The model under review builds one solid part; all positions refer to its coordinate system, in mm. Face numbers are marked on the shaded views. Give positions to 0.01 mm unless a question says otherwise; leave off trailing zeros. Loops run counter-clockwise (first coordinate to the right, second up) from the corner with the lowest first, then second, coordinate; pieces in that order, holes last. Notation, with made-up numbers: M 88.25,-9.75 L 128.25,-9.75 A25 ccw 128.25,20.25 Z; hole C 33.5,53 d10. An arc over 180 degrees is marked long. Return JSON: item names as keys, results as strings.
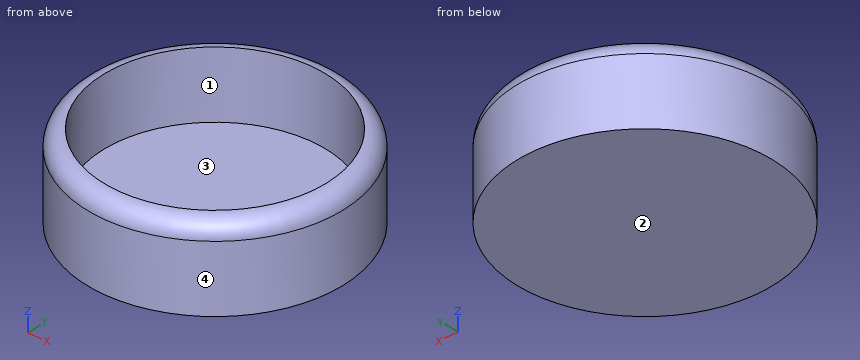
```python
from build123d import *

# Parameters (mm, degrees)
F0_R     = 23
F0_R_2   = 20
F1_DEPTH = 15
F2_R     = 23
F3_DEPTH = 3
F4_R     = 2.99999


# Not quite as in the source:
# - a fillet or chamfer is up to 0.001 mm smaller than in the source, because OpenCascade refuses the exact size


with BuildPart() as f1:
    # F0 (on Top) → F1 (new body)
    with BuildSketch(Plane.XY):
        Circle(F0_R)
        Circle(F0_R_2, mode=Mode.SUBTRACT)
    extrude(amount=F1_DEPTH)

    # F2 (on Top) → F3 (join)
    with BuildSketch(Plane.XY):
        Circle(F2_R)
    extrude(amount=F3_DEPTH)

    # F4 (radius 3 in the source; OpenCascade refuses exactly that, so slightly less here)
    f4_edges = [f1.edges().sort_by_distance(p)[0] for p in [
        (-23, 0, 15),
    ]]
    fillet(f4_edges, radius=F4_R)


solid = f1.part
```
1) Consider section C-C on z = 10.5. Write out the cut boundary in (x, y).
From the geometry:
{"outline": "C 0,0 d46; hole C 0,0 d40"}
2) Consider section D-D on z = 2. Write out the cut boundary in (x, y).
From the geometry:
{"outline": "C 0,0 d46"}
3) The part is to be moulded in two halves that separate along X. For the marked faces 1, 2, 3 and 4, say which applies: released by +X, released by -X, zero draft, split by the parting line, or undercut.
From the geometry:
{"face 1": "undercut", "face 2": "zero draft", "face 3": "undercut", "face 4": "split by the parting line"}
4) Wall thickness on L1, parallel to Y at x = 0, z = 9.5; L2, parallel to Z at x = 15, y = -3; L3, parallel to Y at x = 7.5, z = 9.25: over which ranges is each line inside the solid? List them lowest first. Write a range as from..to.
From the geometry:
{"L1": "-23..-20, 20..23", "L2": "0..3", "L3": "-21.74..-18.54, 18.54..21.74"}
5) Insertion check: pin 1 (2 mm diameter, centred on y = -15.5, z = 5.5, fed in from -X); pin 2 (5 mm diameter, centred on x = -2.5, z = 3.5, fed in from +Y); pin 3 (1 mm diameter, centred on x = 10, y = 10, fed in from -Z); pin 4 (2 mm diameter, centred on x = -9, y = 4, fed in from +Z). Each pin has a flat end and moves straight along its axis. Give the tip position at first contact, or say it passes through.
From the geometry:
{"pin 1": "x = -17.85", "pin 2": "y = 23", "pin 3": "z = 0", "pin 4": "z = 3"}
